Input: dimensioned drawing with shaded views. Units: mm. Origin: part minimum x, y, z. A direction names the side the tool comes from. Round coordinates to 2 decimals unless told otherwise and drop trailing zeros. Order: outer loops, then holes, each group sorted by start corner. A loop starts at its lowest first (then second) coordinate and runs counter-clockwise, first axis right, second up. Notation, with made-up numbers: M 48.25,69 L 75.25,69 A11 cw 75.25,89 Z; hole C -38.75,60 d4. An arc over 180 degrees is marked long. Use one line per item in the form item = value. Start each with the question number.
Q1. Pull-direction query (Y, two-part tool) for the marked faces 1, 2 and 3; classes: pulls with the +Y half, pulls with the -Y half, needs draft (parallel to the pull), parting line crosses it, or undercut.
Q2. Material intervals for probe 1 along Y at (x, z) = (12.7, 11.5); probe 2 along Z at (x, y) = (2.25, 8.5); probe 3 along Y at (x, z) = (12.7, 12.75), sorted ascending.
Q3. Section A-A (y = 10.5). Return the cut outline in (x, z).
Q4. Section B-B (x = 12.7). Return the cut outline in (y, z).
Q5. Section C-C (z = 9). Return the cut outline in (x, y), plus the area to 3 significant figures.
Q6. Reachability of the marked faces 4 and 5 from +Z, -Z, +X, -X, +Y, -Y: full face, straight path, thin tool, end or side. Return the list, or none.
Q7. Section D-D (y = 33.5). Return the cut outline in (x, z).
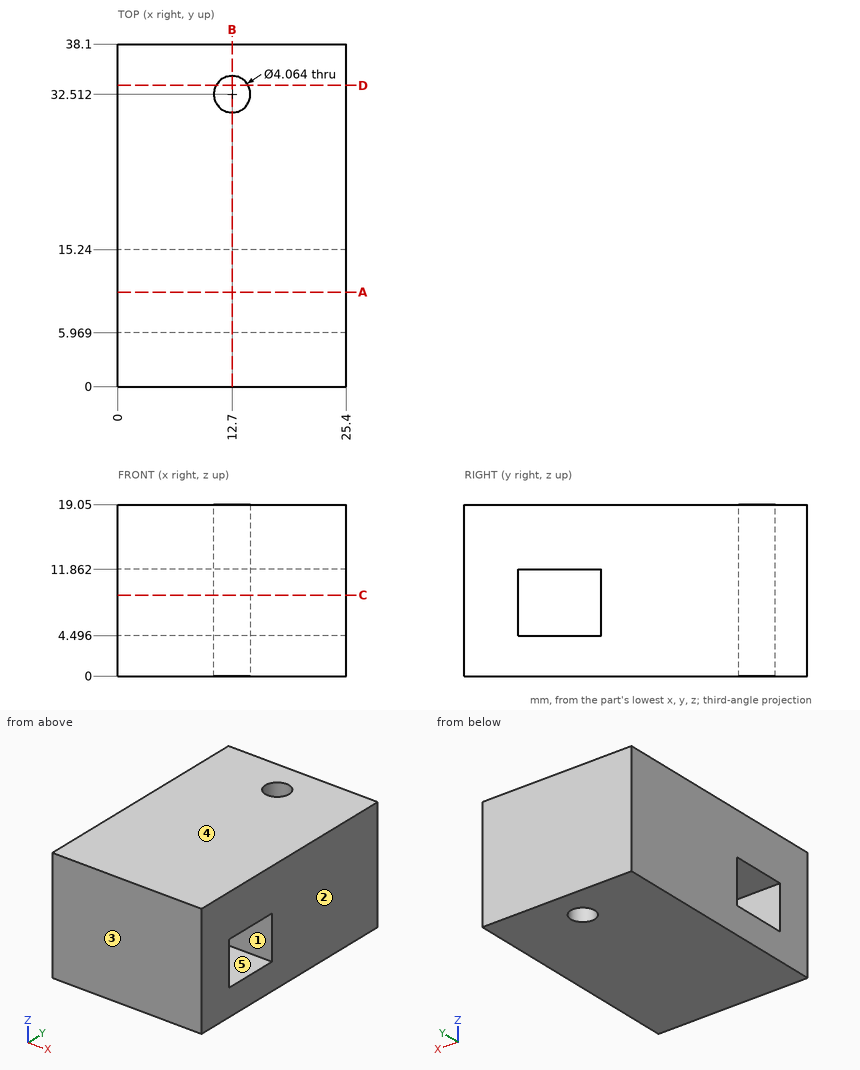
Results list:
q1.face_1 = undercut
q1.face_2 = needs draft
q1.face_3 = pulls with the -Y half
q2.probe_1 = 0 to 5.97, 15.24 to 30.48, 34.54 to 38.1
q2.probe_2 = 0 to 4.5, 11.86 to 19.05
q2.probe_3 = 0 to 30.48, 34.54 to 38.1
q3.outline = M 0,0 L 25.4,0 L 25.4,4.5 L 0,4.5 Z; M 0,11.86 L 25.4,11.86 L 25.4,19.05 L 0,19.05 Z
q4.outline = M 0,0 L 30.48,0 L 30.48,19.05 L 0,19.05 Z; M 34.54,0 L 38.1,0 L 38.1,19.05 L 34.54,19.05 Z; hole M 5.97,4.5 L 15.24,4.5 L 15.24,11.86 L 5.97,11.86 Z
q5.outline = M 0,0 L 25.4,0 L 25.4,5.97 L 0,5.97 Z; M 0,15.24 L 25.4,15.24 L 25.4,38.1 L 0,38.1 Z; hole C 12.7,32.51 d4.06
q5.area = 719 mm2
q6.face_4 = +Z, +X, -X, +Y, -Y
q6.face_5 = +X, -X
q7.outline = M 0,0 L 10.92,0 L 10.92,19.05 L 0,19.05 Z; M 14.48,0 L 25.4,0 L 25.4,19.05 L 14.48,19.05 Z
